Design review of the part built by this model. Coordinates are the model's own, in mm. Face numbers are marked on the shaded views. Coordinates: 2 decimals unless noted, no trailing zeros. Loops run counter-clockwise (first coordinate to the right, second up) from the corner with the lowest first, then second, coordinate; pieces in that order, holes last. Notation, with made-up numbers: (-24, 68.5) - (-15, 68.5) arc R7 cw to (-15, 79.5) - close; hole circle Ø2 at (87, 41). An arc over 180 degrees is marked (long way). Answer in a Markdown table with one row per item. Add a question column.
(1) Clearance check with flat-ended pins moving along their axes: pin 1 (4 mm diameter, centred on y = 15.5, z = -29, fed in from -X); pin 2 (4 mm diameter, centred on x = -50.5, z = 30, fed in from -Y); pin 3 (11 mm diameter, centred on x = -76, z = 12, fed in from +Y); pin 4 (3 mm diameter, centred on y = -59, z = 2, fed in from -X). State where each tip first meets the part, or that it passes through.
(2) We need section C-C, the plane y = 55. Write out the cut boundary in (x, z).
(3) We need section B-B, the plane z = 0. Write out the cut boundary in (x, y), plus the area to 3 significant figures.
(4) The part is to be moulded in two halves that separate along Z. For the marked faces 1, 2 and 3, say which applies: released by +Z, released by -Z, zero draft, split by the parting line, or undercut.
(5) We need section D-D, the plane z = 47. Write out the cut boundary in (x, y), plus the area to 3 significant figures.
(6) To check wall thickness, follow L1, parallel to Y at x = -73, z = 14; L2, parallel to Z at x = -9, y = 34; L3, parallel to Z at x = -47, y = 34.5. State the ranges of each line that lie inside material, in increasing order. Write a range as [from, to].
(7) We need section A-A, the plane x = -47. Write out the cut boundary in (y, z), plus the area to 3 significant figures.
from build123d import *

# Parameters (mm, degrees)
F1_DEPTH = 101.6
F2_DEPTH = 38.1
F3_R     = 3.86409
F4_DEPTH = 25.4
F3_W     = 5.08
F3_H     = 10.050485
F5_DEPTH = 12.7
F6_R     = 2.54
F7_R     = 1.524
F8_DEPTH = 101.6


with BuildPart() as f1:
    # F0 (on Front) → F1 (new body, symmetric)
    with BuildSketch(Plane.XZ):
        with BuildLine():
            ThreePointArc((0, -50.8), (-50.8, 0), (0, 50.8))
            Line((0, 50.8), (0, 57.15))
            ThreePointArc((0, 57.15), (-32.995568, 46.66278), (-53.881537, 19.05))
            ThreePointArc((-53.881537, 19.05), (-57.15, 0), (-53.881537, -19.05))
            ThreePointArc((-53.881537, -19.05), (-32.995568, -46.66278), (0, -57.15))
            Line((0, -57.15), (12.7, -57.15))
            Line((12.7, -57.15), (0, -50.8))
        make_face()
    extrude(amount=F1_DEPTH, both=True)

    # F0 (on Front) → F2 (join, symmetric)
    with BuildSketch(Plane.XZ):
        with BuildLine():
            ThreePointArc((-53.881537, -19.05), (-57.15, 0), (-53.881537, 19.05))
            Line((-53.881537, 19.05), (-67.661227, 19.05))
            Line((-67.661227, 19.05), (-67.661227, -19.05))
            Line((-67.661227, -19.05), (-53.881537, -19.05))
        make_face()
    extrude(amount=F2_DEPTH, both=True)

    # F3 (on face) → F4 (cut)
    with BuildSketch(Plane(origin=(-67.661227, 0, 0), x_dir=(0, -1, 0), z_dir=(-1, 0, 0))):
        with Locations((-26.825511, -9.129036)):
            Circle(F3_R)
        with Locations((26.825511, -9.129036)):
            Circle(F3_R)
    extrude(amount=-F4_DEPTH, mode=Mode.SUBTRACT)

    # F3 (on face) → F5 (join)
    with BuildSketch(Plane(origin=(-67.661227, 0, 0), x_dir=(0, -1, 0), z_dir=(-1, 0, 0))):
        with Locations((-26.67489, 10.3995)):
            Rectangle(F3_W, F3_H)
        with Locations((-16.51489, 10.3995)):
            Rectangle(F3_W, F3_H)
        with Locations((17.42751, 10.3995)):
            Rectangle(F3_W, F3_H)
        with Locations((27.58751, 10.3995)):
            Rectangle(F3_W, F3_H)
    extrude(amount=F5_DEPTH)

    # F6
    f6_edges = [f1.edges().sort_by_distance(p)[0] for p in [
        (-74.011227, 29.21489, 15.424743),
        (-74.011227, 29.21489, 5.374258),
        (-74.011227, 13.97489, 5.374258),
        (-74.011227, 13.97489, 15.424743),
        (-74.011227, -14.88751, 5.374258),
        (-74.011227, -30.12751, 5.374258),
        (-74.011227, -30.12751, 15.424743),
        (-74.011227, -14.88751, 15.424743),
    ]]
    fillet(f6_edges, radius=F6_R)

    # F7 (on face) → F8 (cut)
    with BuildSketch(Plane.XZ.offset(30.12751)):
        with Locations((-75.416334, 10.399501)):
            Circle(F7_R)
    extrude(amount=-F8_DEPTH, mode=Mode.SUBTRACT)


solid = f1.part
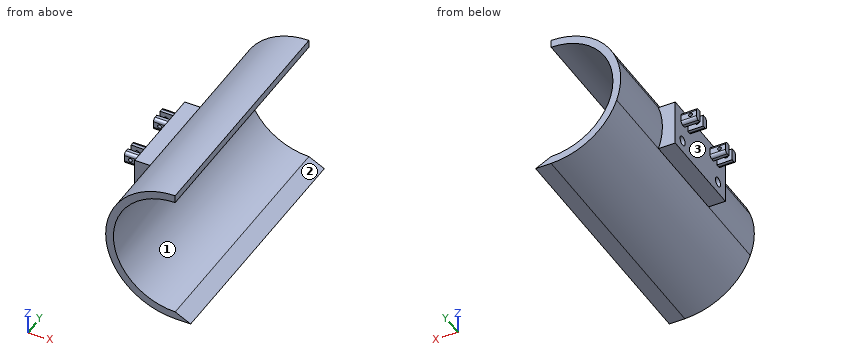
Responses:
| question | item | result |
|---|---|---|
| 1 | pin 1 | stops at x = -50.37 |
| 1 | pin 2 | stops at y = -101.6 |
| 1 | pin 3 | stops at y = 29.21 |
| 1 | pin 4 | stops at x = -57.15 |
| 2 | outline | (-53.88, -19.05) arc R57.15 ccw to (0, -57.15) - (12.7, -57.15) - (0, -50.8) arc R50.8 cw to (0, 50.8) - (0, 57.15) arc R57.15 ccw to (-53.88, 19.05) arc R57.15 ccw to start |
| 3 | outline | (-67.66, -38.1) - (-57.15, -38.1) - (-57.15, -101.6) - (-50.8, -101.6) - (-50.8, 101.6) - (-57.15, 101.6) - (-57.15, 38.1) - (-67.66, 38.1) - close |
| 3 | area | 2,090 mm2 |
| 4 | face 1 | undercut |
| 4 | face 2 | released by +Z |
| 4 | face 3 | zero draft |
| 5 | outline | (-32.51, -101.6) - (-19.28, -101.6) - (-19.28, 101.6) - (-32.51, 101.6) - close |
| 5 | area | 2,690 mm2 |
| 6 | L1 | y = [-29.87, -25.05], [-19.97, -15.15], [14.23, 19.05], [24.13, 28.96] |
| 6 | L2 | z = [-56.44, -50], [50, 56.44] |
| 6 | L3 | z = [-32.51, -19.28], [19.28, 32.51] |
| 7 | outline | (-101.6, -32.51) - (101.6, -32.51) - (101.6, -19.28) - (-101.6, -19.28) - close; (-101.6, 19.28) - (101.6, 19.28) - (101.6, 32.51) - (-101.6, 32.51) - close |
| 7 | area | 5,380 mm2 |
